Verification items for the finished model (mm, model axes). Face numbers are marked on the shaded views. A direction names the side the tool comes from. Give positions to 0.01 mm unless a question says otherwise; leave off trailing zeros. Write each loop counter-clockwise with the first axis right and the second up, starting at its lowest first coordinate (ties: lowest second). Pieces come first, ordered by that corner, then holes. Notation, with made-up numbers: (-32, 64.5) - (-25, 64.5) arc R21 ccw to (-25, 98.5) - close; hole circle Ø1 at (23.25, 82). An arc over 180 degrees is marked (long way). Put each result on its own line as item: value.
Autodesk Inventor part; units mm, degrees
ref_plane "Work Plane9" through (79, -4, -30) normal (0, 0, -1) x (-1, 0, 0)
ref_plane "YZ Plane" through (0, 0, 0) normal (1, 0, 0) x (0, 1, 0)
ref_plane "XZ Plane" through (0, 0, 0) normal (0, 1, 0) x (-1, 0, 0)
sketch "Sketch1" plane through (0, 0, 0) normal (0, 1, 0) x (-1, 0, 0)
  line L0 (80, 30) -> (-80, 30)
  line L1 (-80, 30) -> (-80, -30)
  line L2 (-80, -30) -> (80, -30)
  line L3 (80, -30) -> (80, 30)
  line L4 (80, 30) -> (-80, -30) construction
  line L5 (-80, 30) -> (80, -30) construction
  line L6 (0, -42) -> (0, 42)
  point P0 (0, 0)
  point P1 (-100, -30)
  point P2 (-80, -27)
  dimension "d0" = 160
  dimension "d1" = 60
  dimension "d32" = 20
extrude "Extrusion1" add sketch "Sketch1" along normal blind 3
sketch "Sketch2" plane through (0, 3, 0) normal (0, 1, 0) x (1, 0, 0)
  line L0 (-80, 30) -> (-80, -30)
  line L1 (-80, -30) -> (80, -30)
  line L2 (80, -30) -> (80, 30)
  line L3 (74, -24) -> (-74, -24)
  line L4 (-74, -24) -> (-74, 24)
  line L5 (-74, 24) -> (74, 24)
  line L6 (74, 24) -> (74, -24)
  line L7 (74, -24) -> (-74, 24) construction
  line L8 (-74, -24) -> (74, 24) construction
  line L9 (80, 30) -> (-80, 30)
  point P0 (0, 0)
  dimension "d36" = 148
  dimension "d37" = 48
extrude "Extrusion2" add sketch "Sketch2" along normal blind 24
sketch "Sketch7" plane through (-74, 3, 24) normal (1, 0, 0) x (0, 0, -1)
  circle A0 centre (10, 12) radius 8
  line L0 (54, -3) -> (-6, -3)
  circle A1 centre (10, 12) radius 10
  line L1 (0, 12) -> (0, 0)
  line L2 (0, 12) -> (20, 12)
  line L3 (20, 12) -> (20, 0)
  line L4 (-6, -3) -> (-6, 24)
  line L5 (0, 0) -> (20, 0)
  line L6 (10, 22) -> (0, 22)
  line L7 (0, 0) -> (0, 24)
  line L8 (0, 12) -> (0, 22)
  point P0 (24, -3)
  point P1 (54, -3)
  dimension "MotorDiameter" = 16
  dimension "d18" = 15
  dimension "d20" = 2
  dimension "d40" = 20
  dimension "d62" = 10
extrude "Extrusion5" add sketch "Sketch7" along normal blind 11.25 contours L2 A1 A0 | A0 L2 A1 | L3 L5 L1 A1 | L7 L6 A1
sketch "Sketch8" plane through (-62.75, 3, 24) normal (1, 0, 0) x (0, 0, -1)
  arc A0 (20, 12) -> (10, 22) centre (10, 12) ccw
  circle A1 centre (10, 12) radius 8
  line L0 (0, 0) -> (0, 22)
  line L1 (20, 0) -> (0, 0)
  line L2 (20, 0) -> (20, 12)
  circle A2 centre (10, 12) radius 7.75
  line L3 (10, 22) -> (0, 22)
  line L4 (0, 0) -> (0, 22)
  line L5 (4, 7.0946) -> (4, 17.2915)
  line L6 (10, 22) -> (0, 22)
  line L7 (16, 7.0946) -> (16, 17.2915)
  line L8 (16, 17.2915) -> (18.4853, 17.2915)
  arc A3 (20, 12) -> (10, 22) centre (10, 12) ccw
  line L9 (4, 17.2915) -> (0, 17.2915)
  point P0 (24, -3)
  point P1 (4, 27)
  point P2 (4, 16.9054)
  point P3 (16, 16.9054)
  dimension "d55" = 15.5
  dimension "d63" = 12
  dimension "d64" = 6
extrude "Extrusion6" add sketch "Sketch8" along normal blind 20 contours L2 L1 L0 L9 A1 L8 A0 | A1 L5 A2 L7 | A2 L7 | L5 A2 picked at (9.114, 4.2488)
sketch "Sketch9" plane through (-74, 20, 20) normal (1, 0, 0) x (0, 0, -1)
  circle A0 centre (6, -5) radius 3.5
  line L0 (50, -20) -> (-10, -20)
  line L1 (-10, -20) -> (-10, 7)
  point P0 (20, -20)
  point P1 (44, -20)
  dimension "d27" = 7
  dimension "d28" = 15
  dimension "d41" = 16
extrude "Extrusion7" cut sketch "Sketch9" against normal up to surface (6 mm away)
mirror "Mirror2" about plane through (0, 0, 0) normal (1, 0, 0) of "Extrusion7", "Extrusion6", "Extrusion5"
sketch "Sketch15" plane through (80, 0, 30) normal (1, 0, 0) x (0, 0, -1)
  line L0 (60, 27) -> (0, 27)
  circle A0 centre (16, 15) radius 3.5
  line L1 (0, 0) -> (60, 0)
  line L2 (60, 0) -> (60, 27)
  line L3 (0, 27) -> (60, 27)
  line L4 (0, 0) -> (0, 27)
  line L5 (60, 0) -> (60, 27)
  line L6 (120.0188, 15.0047) -> (60, 0)
  line L7 (60, 0) -> (60, 27)
  line L8 (60, 0) -> (60, 30)
  line L9 (60, 15) -> (120, 15)
  line L10 (60, 30) -> (120, 15)
  point P0 (30, 0)
  dimension "d104" = 30
  dimension "d105" = 15
  dimension "d106" = 60
extrude "Extrusion18" add sketch "Sketch15" against normal up to surface (160 mm away) contours L8 L10 L9 L2 | L9 L6 L2
ref_plane "Work Plane9" through (79, -4, -30) normal (0, 0, -1) x (-1, 0, 0)
sketch "Sketch23" plane through (79, -4, -30) normal (0, 0, -1) x (-1, 0, 0)
  line L0 (-1, 34) -> (-21, 19)
  line L1 (-21, 19) -> (-1, 19)
  line L2 (-21, 19) -> (-1, 4)
  line L3 (-1, 31) -> (159, 31)
  line L4 (-1, 34) -> (-1, 31)
  line L5 (-1, 34) -> (159, 34)
  line L6 (159, 34) -> (159, 31)
  line L7 (159, 4) -> (-1, 4)
  line L8 (-1, 4) -> (-1, 31)
  line L9 (159, 31) -> (-1, 31)
  line L10 (159, 4) -> (159, 31)
  point P0 (79, 4)
  dimension "d97" = 20
  dimension "d108" = 15
extrude "Extrusion19" add sketch "Sketch23" along normal blind 60 contours L4 L8 L1 L0 | L1 L8 L2
ref_plane "Work Plane4" through (100, 15, -30) normal (-0.5883, -0.7845, 0.1961) x (-0.8, 0.6, 0)
sketch "Sketch24" plane through (100, 15, -30) normal (-0.5883, -0.7845, 0.1961) x (-0.8, 0.6, 0)
  line L0 (-89.1969, -73.3175) -> (145.8797, -73.3175)
  line L1 (145.8797, -73.3175) -> (145.8797, 67.3582)
  line L2 (145.8797, 67.3582) -> (-89.1969, 67.3582)
  line L3 (-89.1969, 67.3582) -> (-89.1969, -73.3175)
  point P0 (71, -15.2971)
extrude "Extrusion20" cut sketch "Sketch24" against normal blind 60
ref_plane "Work Plane5" through (80, 15, -90) normal (0.5883, -0.7845, -0.1961) x (0.3162, 0, 0.9487)
sketch "Sketch25" plane through (80, 15, -90) normal (0.5883, -0.7845, -0.1961) x (0.3162, 0, 0.9487)
  line L0 (-115.6054, 99.2741) -> (196.6383, 99.2741)
  line L1 (196.6383, 99.2741) -> (196.6383, -110.1424)
  line L2 (196.6383, -110.1424) -> (-115.6054, -110.1424)
  line L3 (-115.6054, -110.1424) -> (-115.6054, 99.2741)
  point P0 (60.0833, 91.1655)
extrude "Extrusion21" cut sketch "Sketch25" along normal blind 60
mirror "Mirror10" about plane through (0, 0, 0) normal (1, 0, 0) of "Extrusion19", "Extrusion20", "Extrusion21"
sketch "Sketch26" plane through (0, 27, 0) normal (0, 1, 0) x (1, 0, 0)
  line L0 (-80, 30) -> (-80, -30)
  line L1 (-80, -30) -> (80, -30)
  line L2 (80, -30) -> (80, 30)
  line L3 (80, 30) -> (-80, 30)
  line L4 (-74, 24) -> (74, 24)
  line L5 (74, 24) -> (74, -24)
  line L6 (74, -24) -> (-74, -24)
  line L7 (-74, -24) -> (-74, 24)
  point P0 (0, 0)
extrude "Extrusion22" add sketch "Sketch26" along normal blind 1.4125
sketch "Sketch27" plane through (0, 28.4125, 0) normal (0, 1, 0) x (1, 0, 0)
  line L0 (-80, 30) -> (-80, -30)
  line L1 (-80, -30) -> (80, -30)
  line L2 (80, -30) -> (80, 30)
  line L3 (-80, 30) -> (80, 30)
  line L4 (-74, -24) -> (-74, 24)
  line L5 (-74, 24) -> (74, 24)
  line L6 (74, 24) -> (74, -24)
  line L7 (74, -24) -> (-74, -24)
  line L8 (80, -30) -> (80, 30)
  line L9 (80, -27) -> (-80, -27)
  line L10 (-80, 30) -> (-80, -30)
  line L11 (80, 27) -> (-80, 27)
  line L12 (-80, -30) -> (80, -30)
  line L13 (77, -30) -> (77, 30)
  circle A0 centre (63, -27) radius 1.45
  circle A1 centre (77, 27) radius 1.45
  line L14 (0, 114) -> (0, -54)
  circle A2 centre (-63, -27) radius 1.45
  circle A3 centre (-77, 27) radius 1.45
  point P0 (0, 0)
  dimension "d111" = 3
  dimension "d112" = 3
  dimension "d113" = 3
  dimension "d114" = 2.9
  dimension "d115" = 17
  dimension "d116" = 2.9
extrude "Extrusion23" cut sketch "Sketch27" against normal blind 7 contours A3 L11 | L11 A3 | A2 L9 | L9 A2 | A1 L11 L13 | L13 L11 A1 | L11 L13 A1 | L11 A1 L13 | A0 L9 | L9 A0
ref_plane "Work Plane7" through (-100, 15, -30) normal (-0.5883, 0.7845, -0.1961) x (0.8, 0.6, 0)
ref_plane "Work Plane8" through (-80, 15, -90) normal (0.5883, 0.7845, 0.1961) x (-0.3162, 0, 0.9487)
equation "\"d0\" = Width"
equation "\"d1\" = Length"
equation "\"d2\" = BaseWallThickness"
equation "\"d36\" = Width - 2 * SideWallThickness"
equation "\"d37\" = Length - 2 * SideWallThickness"
equation "\"d5\" = Height - 2 * BaseWallThickness"
equation "\"d18\" = DriveMotorHeight"
equation "\"d20\" = DriveMotorMountThickness"
equation "\"d28\" = DriveMotorHeight"
equation "\"d41\" = SideWallThickness + DriveMotorMountThickness + 0.5 * MotorDiameter"
equation "\"d104\" = Height"
equation "\"d105\" = 0.5 * Height"
equation "\"d106\" = WedgeLength"
equation "\"d97\" = SideTriangleWidth"
equation "\"d98\" = WedgeLength"
equation "\"d100\" = WedgeLength"
equation "\"d102\" = WedgeLength"
equation "\"SideWallThickness\" = 6"
equation "\"BaseWallThickness\" = 3"
equation "\"Width\" = 160"
equation "\"Length\" = 60"
equation "\"Height\" = 30"
equation "\"DriveMotorHeight\" = 0.5 * Height"
equation "\"DriveMotorMountThickness\" = 2"
equation "\"WedgeLength\" = 60"
equation "\"SideTriangleWidth\" = 20"
equation "\"ScrewHoleDia\" = 2.9"
equation "\"ScrewDepth\" = 7"
properties part number "BodyWedgeV3" material "Thermoplastic Resin"
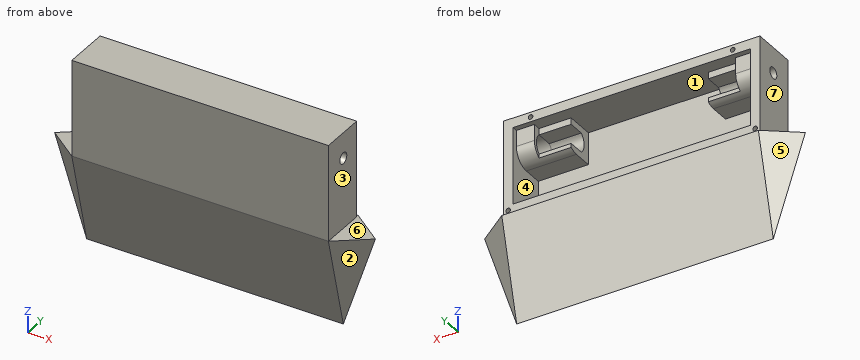
Q1. Section check D-D, the plane x = 57. Record the cut outline in (y, z), plus the area to 3 significant figures.
Answers follow:
outline: (0, -30) - (15, -90) - (30, -30) - (28.41, -30) - (28.41, -24) - (3, -24) - (3, 4) - (15, 4) arc R10 ccw to (20.29, 5.51) - (20.29, 8) - (10.09, 8) arc R7.75 cw to (10.09, 20) - (20.29, 20) - (20.29, 24) - (28.41, 24) - (28.41, 30) - (0, 30) - close
area: 1,580 mm2
Q2. Section check A-A, the plane x = -70.5. Record the cut outline in (y, z), plus the area to 3 significant figures.
Answers follow:
outline: (0, -30) - (15, -90) - (30, -30) - (28.41, -30) - (28.41, -24) - (3, -24) - (3, 4) - (15, 4) arc R10 ccw to (25, 14) - (25, 24) - (28.41, 24) - (28.41, 30) - (0, 30) - close; hole circle Ø16 at (15, 14)
area: 1,600 mm2
Q3. Section check C-C, the plane z = 2. Record the cut outline in (x, y), plus the area to 3 significant figures.
Answers follow:
outline: (-80, 0) - (80, 0) - (80, 28.41) - (74, 28.41) - (74, 3) - (-74, 3) - (-74, 28.41) - (-80, 28.41) - close
area: 785 mm2
Q4. Set-up check for the marked faces 4, 5, 6 and 7: record each of +Z, -Z, +X, -X, +Y, -Y from which the full face is reachable in a straight line by a thin tool's end or side.
Answers follow:
face 4: +Y
face 5: -Z, -X, +Y
face 6: +Z, +Y
face 7: +Z, -X, +Y, -Y
Q5. Release check for a two-part mould opening along Z. For the marked faces 1, 2 and 3 record: released by +Z, released by -Z, zero draft, split by the parting line, or undercut.
Answers follow:
face 1: undercut
face 2: released by -Z
face 3: zero draft
Q6. Go/stop test with flat-tipped pins: pin 1 Ø4 at (y, z) = (23, 18) entering from +X; pin 2 Ø4 at (y, z) = (11.5, 12) entering from -X; pin 3 Ø3 at (x, z) = (50, -58.5) entering from -Y. Record where each tip stops, or that it passes through.
Answers follow:
pin 1: stops at x = 80
pin 2: stops at x = -80
pin 3: stops at y = 6.75
Q7. Scan lines: line 1 along X through (y, z) = (26, -27); line 2 along X through (y, z) = (14.5, 19); line 3 along X through (y, z) = (25.5, 27). Record each from-to range of solid material in increasing order.
Answers follow:
line 1: x = -80 to -78.45, -75.55 to 75.55, 78.45 to 80
line 2: x = -80 to -74, 74 to 80
line 3: x = -80 to -64.45, -61.55 to 61.55, 64.45 to 80
Q8. Section check B-B, the plane x = -15.5. Record the cut outline in (y, z).
Answers follow:
outline: (0, -30) - (15, -90) - (30, -30) - (28.41, -30) - (28.41, -24) - (3, -24) - (3, 24) - (28.41, 24) - (28.41, 30) - (0, 30) - close
